CAD build for the part. Positions are in the model's coordinates, mm. A direction names the side the tool comes from. Coordinates: 2 decimals unless noted, no trailing zeros. Loops run counter-clockwise (first coordinate to the right, second up) from the corner with the lowest first, then second, coordinate; pieces in that order, holes last. Notation, with made-up numbers: (23, 16) -> (41, 16) arc R9 ccw to (41, 24) -> close; hole circle Ø2 at (-1, 74.5). An arc over 180 degrees is marked (long way). Write each question's results on one line, items separated by ' | '.
from build123d import *

# Parameters (mm, degrees)
SKETCH1_W                    = 35
SKETCH1_H                    = 12
BASE_FLANGE1_DEPTH           = 2
EDGE_FLANGE1_STRIP_W         = 12
EDGE_FLANGE1_STRIP_H         = 2
EDGE_FLANGE1_STRIP_CUT_DEPTH = 35
EDGE_FLANGE1_DEPTH           = 35
FILLET1_R                    = 2
SKETCH9_R                    = 1
CUT_EXTRUDE1_DEPTH           = 10
SKETCH10_R                   = 3
SKETCH10_R_2                 = 1.5
SKETCH10_R_3                 = 1
CUT_EXTRUDE2_DEPTH           = 10
SKETCH11_R                   = 1.6
CUT_EXTRUDE3_DEPTH           = 10


# Sheet-metal steps are written as plain solids
with BuildPart() as part:
    # Sketch1 → Base-Flange1 (new body)
    with BuildSketch(Plane.XY):
        Rectangle(SKETCH1_W, SKETCH1_H)
    extrude(amount=-BASE_FLANGE1_DEPTH)

    # Edge-Flange1 strip (across the edge) → Edge-Flange1 strip cut (cut)
    with BuildSketch(Plane(origin=(-17.5, -6, 0), x_dir=(0, 1, 0), z_dir=(1, 0, 0))):
        with Locations((-2, -1)):
            Rectangle(EDGE_FLANGE1_STRIP_W, EDGE_FLANGE1_STRIP_H)
    extrude(amount=EDGE_FLANGE1_STRIP_CUT_DEPTH, mode=Mode.SUBTRACT)

    # Edge-Flange1 section (across the edge) → Edge-Flange1 (add)
    with BuildSketch(Plane(origin=(-17.5, -6, 0), x_dir=(0, 1, 0), z_dir=(1, 0, 0))):
        with BuildLine():
            Line((0, 2), (0, 22))
            Line((0, 22), (2, 22))
            Line((2, 22), (2, 2))
            ThreePointArc((2, 2), (2.585786438, 0.585786438), (4, 0))
            Line((4, 0), (4, -2))
            ThreePointArc((4, -2), (1.171572875, -0.828427125), (0, 2))
        make_face()
    extrude(amount=EDGE_FLANGE1_DEPTH)

    # Fillet1
    fillet1_edges = [part.edges().sort_by_distance(p)[0] for p in [
        (-17.5, -5, 22),
        (17.5, -5, 22),
        (-17.5, 6, -1),
        (17.5, 6, -1),
    ]]
    fillet(fillet1_edges, radius=FILLET1_R)

    # Sketch9 → Cut-Extrude1 (cut)
    with BuildSketch(Plane(origin=(0, 0, -2), x_dir=(-1, 0, 0), z_dir=(0, 0, -1))):
        with Locations((4, 2)):
            Circle(SKETCH9_R)
        with Locations((12, 2)):
            Circle(SKETCH9_R)
        with Locations(Location((-12, 2, 0), (0, 0, 180))):
            Circle(SKETCH9_R)
        with Locations(Location((-4, 2, 0), (0, 0, 180))):
            Circle(SKETCH9_R)
    extrude(amount=-CUT_EXTRUDE1_DEPTH, mode=Mode.SUBTRACT)

    # Sketch10 → Cut-Extrude2 (cut)
    with BuildSketch(Plane.XZ.offset(6)):
        with Locations(Location((0, 11, 0), (0, 0, 270))):
            Circle(SKETCH10_R)
        with Locations(Location((-7, 11, 0), (0, 0, 270))):
            Circle(SKETCH10_R_2)
        with Locations(Location((-15, 5, 0), (0, 0, 270))):
            Circle(SKETCH10_R_2)
        with Locations(Location((-15, 17, 0), (0, 0, 270))):
            Circle(SKETCH10_R_3)
        with Locations(Location((-4.949747468, 15.949747468, 0), (0, 0, 270))):
            Circle(SKETCH10_R_3)
        with Locations(Location((-4.949747468, 6.050252532, 0), (0, 0, 270))):
            Circle(SKETCH10_R_3)
        with Locations(Location((0, 18, 0), (0, 0, 270))):
            Circle(SKETCH10_R_2)
        with Locations(Location((15, 17, 0), (0, 0, 90))):
            Circle(SKETCH10_R_3)
        with Locations(Location((15, 5, 0), (0, 0, 90))):
            Circle(SKETCH10_R_2)
        with Locations(Location((4.949747468, 6.050252532, 0), (0, 0, 90))):
            Circle(SKETCH10_R_3)
        with Locations(Location((7, 11, 0), (0, 0, 90))):
            Circle(SKETCH10_R_2)
        with Locations(Location((4.949747468, 15.949747468, 0), (0, 0, 90))):
            Circle(SKETCH10_R_3)
    extrude(amount=-CUT_EXTRUDE2_DEPTH, mode=Mode.SUBTRACT)

    # Sketch11 → Cut-Extrude3 (cut)
    with BuildSketch(Plane.XY):
        with Locations((-10.205953252, 5.743869118)):
            Circle(SKETCH11_R)
        with Locations((3.631753083, 6.323821502)):
            Circle(SKETCH11_R)
    extrude(amount=-CUT_EXTRUDE3_DEPTH, mode=Mode.SUBTRACT)


solid = part.part
1) Slice it at B-B (y = 2). Write the cut outline in (x, z), then the cut area to 3 significant figures.
Outcome:
outline: (-17.5, -2) -> (-13, -2) -> (-13, 0) -> (-17.5, 0) -> close; (-11, -2) -> (-5, -2) -> (-5, 0) -> (-11, 0) -> close; (-3, -2) -> (3, -2) -> (3, 0) -> (-3, 0) -> close; (5, -2) -> (11, -2) -> (11, 0) -> (5, 0) -> close; (13, -2) -> (17.5, -2) -> (17.5, 0) -> (13, 0) -> close | area: 54.0 mm^2
2) Pin check, flat tips, straight feed: pin 1 (10 mm diameter, centred on x = 9, z = 7, fed in from +Y); pin 2 (1 mm diameter, centred on x = 12, y = -5, fed in from -Z); pin 3 (3 mm diameter, centred on x = 12, y = 2, fed in from +Z). Stop position of each tip, or through.
Outcome:
pin 1: stops at y = -4 | pin 2: stops at z = -1.12 | pin 3: stops at z = 0
3) Slice it at C-C (z = 11). Write the cut outline in (x, y).
Outcome:
outline: (-17.5, -6) -> (-8.5, -6) -> (-8.5, -4) -> (-17.5, -4) -> close; (-5.5, -6) -> (-3, -6) -> (-3, -4) -> (-5.5, -4) -> close; (3, -6) -> (5.5, -6) -> (5.5, -4) -> (3, -4) -> close; (8.5, -6) -> (17.5, -6) -> (17.5, -4) -> (8.5, -4) -> close
4) Slice it at A-A (x = -15). Write the cut outline in (y, z), then the cut area to 3 significant figures.
Outcome:
outline: (-6, 2) arc R4 ccw to (-2, -2) -> (6, -2) -> (6, 0) -> (-2, 0) arc R2 cw to (-4, 2) -> (-4, 3.5) -> (-6, 3.5) -> close; (-6, 6.5) -> (-4, 6.5) -> (-4, 16) -> (-6, 16) -> close; (-6, 18) -> (-4, 18) -> (-4, 22) -> (-6, 22) -> close | area: 55.4 mm^2
5) Slice it at D-D (x = -7). Write the cut outline in (y, z), then the cut area to 3 significant figures.
Outcome:
outline: (-6, 2) arc R4 ccw to (-2, -2) -> (6, -2) -> (6, 0) -> (-2, 0) arc R2 cw to (-4, 2) -> (-4, 9.5) -> (-6, 9.5) -> close; (-6, 12.5) -> (-4, 12.5) -> (-4, 22) -> (-6, 22) -> close | area: 59.4 mm^2
6) Which spindle directions (+Z, -Z, +X, -X, +Y, -Y) get a long thin tool onto all of the face, cutting with end or side? Do faces 1 (the flat face through (-14, 6, -1)), 2 (the flat face through (0, 2, 0)). Say none if no direction does.
Outcome:
face 1: +Z, -Z, +X, -X, +Y | face 2: +Z, +X, -X, +Y
7) Two-plate mould, pull along Z, no slides. Class faces 3 (the cylindrical face through (-5.56, -5.01, 6.84)), 4 (the flat face through (0, 2, -2)), 5 (the cylindrical face through (3, 2, -1)): pulls with the +Z half, pulls with the -Z half, needs draft (parallel to the pull), parting line crosses it, or undercut.
Outcome:
face 3: undercut | face 4: pulls with the -Z half | face 5: needs draft
8) Drill centre lines: L1, parallel to X at y = -4.4, z = 5; L2, parallel to X at y = -5, z = 11; L3, parallel to Y at x = -10, z = 15. Where is each one in solid material? Low to high. Write a range as from..to.
Outcome:
L1: x = -17.5..-16.5, -13.5..13.5, 16.5..17.5 | L2: x = -17.5..-8.5, -5.5..-3, 3..5.5, 8.5..17.5 | L3: y = -6..-4
